Could you check a few things on this model? Use its own coordinates, in mm. A direction names the side the tool comes from. Coordinates: 2 decimals unless noted, no trailing zeros. Loops run counter-clockwise (first coordinate to the right, second up) from the corner with the lowest first, then second, coordinate; pieces in that order, holes last.
from build123d import *

# Parameters (mm, degrees)
SKETCH1_R           = 4
SKETCH1_R_2         = 1.6
BOSS_EXTRUDE1_DEPTH = 3
SKETCH2_W           = 26.2
SKETCH2_H           = 29.8
SKETCH2_R           = 2
SKETCH2_R_2         = 5
BOSS_EXTRUDE2_DEPTH = 3
FILLET1_R           = 2


with BuildPart() as part:
    # Sketch1 → Boss-Extrude1 (new body)
    with BuildSketch(Plane.XY):
        with BuildLine():
            Line((-13.1, 20.4), (-13.1, 0))
            Line((-13.1, 0), (13.1, 0))
            Line((13.1, 0), (13.1, 20.4))
            ThreePointArc((13.1, 20.4), (0, 33.5), (-13.1, 20.4))
        make_face()
        with Locations((0, 20.4)):
            Circle(SKETCH1_R, mode=Mode.SUBTRACT)
        with Locations((-8.5, 20.4)):
            Circle(SKETCH1_R_2, mode=Mode.SUBTRACT)
        with Locations((8.5, 20.4)):
            Circle(SKETCH1_R_2, mode=Mode.SUBTRACT)
    extrude(amount=BOSS_EXTRUDE1_DEPTH)

    # Sketch2 → Boss-Extrude2 (add)
    with BuildSketch(Plane.XZ):
        with Locations((0, 17.9)):
            Rectangle(SKETCH2_W, SKETCH2_H)
        with Locations((8, 24.9)):
            Circle(SKETCH2_R, mode=Mode.SUBTRACT)
        with Locations((8, 10.9)):
            Circle(SKETCH2_R, mode=Mode.SUBTRACT)
        with Locations((-8, 10.9)):
            Circle(SKETCH2_R, mode=Mode.SUBTRACT)
        with Locations((-8, 24.9)):
            Circle(SKETCH2_R, mode=Mode.SUBTRACT)
        with Locations((0, 17.9)):
            Circle(SKETCH2_R_2, mode=Mode.SUBTRACT)
    extrude(amount=-BOSS_EXTRUDE2_DEPTH)

    # Fillet1
    fillet1_edges = [part.edges().sort_by_distance(p)[0] for p in [
        (13.1, 1.5, 32.8),
        (0, 3, 3),
        (-13.1, 1.5, 32.8),
        (0, 0, 0),
    ]]
    fillet(fillet1_edges, radius=FILLET1_R)


solid = part.part
(1) We'd pull the mould along Z, two halves only. Please class faces 3 (the face through (-8.26, 1.479, 26.883)), 4 (the face through (0.18, 0.6, 0.57)), 5 (the face through (13.1, 2.6, 9.6)): +Z half, -Z half, draft (parallel to the pull), parting line (faces both ways), or undercut.
Answers:
face 3: undercut
face 4: -Z half
face 5: draft
(2) Imagine slicing it at B-B, the plane z = 10.9. Write out the boundary of the cut face in (x, y).
Answers:
outline: (-13.1, 0) - (-10, 0) - (-10, 3) - (-13.1, 3) - close; (-6, 0) - (6, 0) - (6, 3) - (-6, 3) - close; (10, 0) - (13.1, 0) - (13.1, 3) - (10, 3) - close
(3) Imagine slicing it at C-C, the plane x = -8.5. Write out the boundary of the cut face in (y, z), and give its area (3 significant figures).
Answers:
outline: (0, 2) arc R2 ccw to (2, 0) - (18.8, 0) - (18.8, 3) - (5, 3) arc R2 cw to (3, 5) - (3, 8.96) - (0, 8.96) - close; (0, 12.84) - (3, 12.84) - (3, 22.96) - (0, 22.96) - close; (0, 26.84) - (3, 26.84) - (3, 32.8) - (0, 32.8) - close; (22, 0) - (30.37, 0) - (30.37, 3) - (22, 3) - close
area: 148 mm2
(4) Imagine slicing it at D-D, the plane z = 22. Write out the boundary of the cut face in (x, y).
Answers:
outline: (-13.1, 0) - (-2.86, 0) - (-2.86, 3) - (-13.1, 3) - close; (2.86, 0) - (13.1, 0) - (13.1, 3) - (2.86, 3) - close
(5) Imagine slicing it at A-A, the plane x = 0. Write out the boundary of the cut face in (y, z), and give its area (3 significant figures).
Answers:
outline: (0, 2) arc R2 ccw to (2, 0) - (16.4, 0) - (16.4, 3) - (5, 3) arc R2 cw to (3, 5) - (3, 12.9) - (0, 12.9) - close; (0, 22.9) - (3, 22.9) - (3, 32.8) - (0, 32.8) - close; (24.4, 0) - (33.5, 0) - (33.5, 3) - (24.4, 3) - close
area: 136 mm2
(6) Which directions (+Z, -Z, +X, -X, +Y, -Y) give clear straight access to the entire face, cutting with the end or side of a thin tool? Please do faces 1 (the face through (0, 16, 3)), 2 (the face through (-13.1, 2.6, 9.6)).
Answers:
face 1: +Z, +X, -X, +Y
face 2: +Z, -Z, -X, +Y, -Y
(7) I need wall thicknesses on probe 1 along X at (y, z) = (20, 2); probe 2 along X at (y, z) = (1, 10); probe 3 along Z at (x, y) = (-0.5, 32). Which ranges of each line are inside material? Lowest first, please.
Answers:
probe 1: x = -13.1 to -10.05, -6.95 to -3.98, 3.98 to 6.95, 10.05 to 13.1
probe 2: x = -13.1 to -9.79, -6.21 to 6.21, 9.79 to 13.1
probe 3: z = 0 to 3
(8) For pin 1 (4.5 mm diameter, centred on x = -8, z = 10.9, fed in from +Y); pin 2 (8 mm diameter, centred on x = 5.5, y = 16.5, fed in from +Z), each with a flat end and sliding along its axis, tell me the tip position at first contact or that it passes through.
Answers:
pin 1: stops at y = 3
pin 2: stops at z = 3
